```python
from build123d import *

# Parameters (mm, degrees)
F0_W     = 38.1
F0_H     = 127
F3_R     = 6.35
F4_DEPTH = 12.7
F5_COUNT = 8


with BuildPart() as f1:
    # F0 (on Front) → F1 (revolve)
    with BuildSketch(Plane.XZ):
        with Locations((-19.05, 0)):
            Rectangle(F0_W, F0_H)
    revolve(axis=Axis((0, 0, 0), (0, 0, -1)))


with BuildPart() as f4:
    # F3 (on offset) → F4 (new body)
    with BuildSketch(Plane.XZ.offset(38.1)):
        Circle(F3_R)
    extrude(amount=F4_DEPTH)


with BuildPart() as f5_1:
    # F5: instance of F4
    add(f4.part.rotate(Axis((0, 0, 63.5), (0, 0, -1)), 1 * 360 / F5_COUNT))


with BuildPart() as f5_2:
    # F5: instance of F4
    add(f4.part.rotate(Axis((0, 0, 63.5), (0, 0, -1)), 2 * 360 / F5_COUNT))


with BuildPart() as f5_3:
    # F5: instance of F4
    add(f4.part.rotate(Axis((0, 0, 63.5), (0, 0, -1)), 3 * 360 / F5_COUNT))


with BuildPart() as f5_4:
    # F5: instance of F4
    add(f4.part.rotate(Axis((0, 0, 63.5), (0, 0, -1)), 4 * 360 / F5_COUNT))


with BuildPart() as f5_5:
    # F5: instance of F4
    add(f4.part.rotate(Axis((0, 0, 63.5), (0, 0, -1)), 5 * 360 / F5_COUNT))


with BuildPart() as f5_6:
    # F5: instance of F4
    add(f4.part.rotate(Axis((0, 0, 63.5), (0, 0, -1)), 6 * 360 / F5_COUNT))


with BuildPart() as f5_7:
    # F5: instance of F4
    add(f4.part.rotate(Axis((0, 0, 63.5), (0, 0, -1)), 7 * 360 / F5_COUNT))


with BuildPart() as f1_1:
    add(f1.part)

    # F6: cut F4, F5_1, F5_2, F5_3, F5_4, F5_5, F5_6, F5_7
    add(f4.part, mode=Mode.SUBTRACT)
    add(f5_1.part, mode=Mode.SUBTRACT)
    add(f5_2.part, mode=Mode.SUBTRACT)
    add(f5_3.part, mode=Mode.SUBTRACT)
    add(f5_4.part, mode=Mode.SUBTRACT)
    add(f5_5.part, mode=Mode.SUBTRACT)
    add(f5_6.part, mode=Mode.SUBTRACT)
    add(f5_7.part, mode=Mode.SUBTRACT)


solid = f1_1.part
```
Here's how the part is built. I have some questions about the finished solid (model axes, mm). Round coordinates to 2 decimals unless told otherwise and drop trailing zeros. Loops run counter-clockwise (first coordinate to the right, second up) from the corner with the lowest first, then second, coordinate; pieces in that order, holes last. Notation, with made-up numbers: (57, -37) -> (110, -37) arc R19 ccw to (110, -12) -> close; hole circle Ø2 at (80, 40.5). An arc over 180 degrees is marked (long way). Answer as CSV lines item,"result". Start each with the question number.
1. I'm going to push flat-ended pins straight in: P1, Ø10, axis at x = 16, z = 42, coming from the -Y side; P2, Ø1, axis at y = -26.5, z = 46.5, coming from the +X side; P3, Ø10, axis at x = 21.5, z = 10.5, coming from the +Y side. Where does each tip first touch, or does it pass through?
2. I need wall thicknesses on probe 1 along X at (y, z) = (-0.5, -15); probe 2 along X at (y, z) = (31.5, 44.5); probe 3 along Y at (x, z) = (30.5, -30.5). Which ranges of each line are inside material? Lowest first, please. Write a range as from..to.
3. Imagine slicing it at A-A on z = 42. Write out the boundary of the cut face in (x, y).
4. Imagine slicing it at B-B on x = -10.5. Write out the boundary of the cut face in (y, z).
5. Imagine slicing it at C-C on y = 19. Write out the boundary of the cut face in (x, z), plus the area to 3 significant figures.
Solution:
1,P1,"y = -36.48"
1,P2,"x = 27.85"
1,P3,"y = 34.34"
2,probe 1,"-38.1..38.1"
2,probe 2,"-21.43..21.43"
2,probe 3,"-22.83..22.83"
3,outline,"circle Ø76.2 at (0, 0)"
4,outline,"(-36.62, -63.5) -> (36.62, -63.5) -> (36.62, 63.5) -> (-36.62, 63.5) -> close"
5,outline,"(-33.02, -63.5) -> (33.02, -63.5) -> (33.02, 63.5) -> (-33.02, 63.5) -> close"
5,area,"8,390 mm²"
